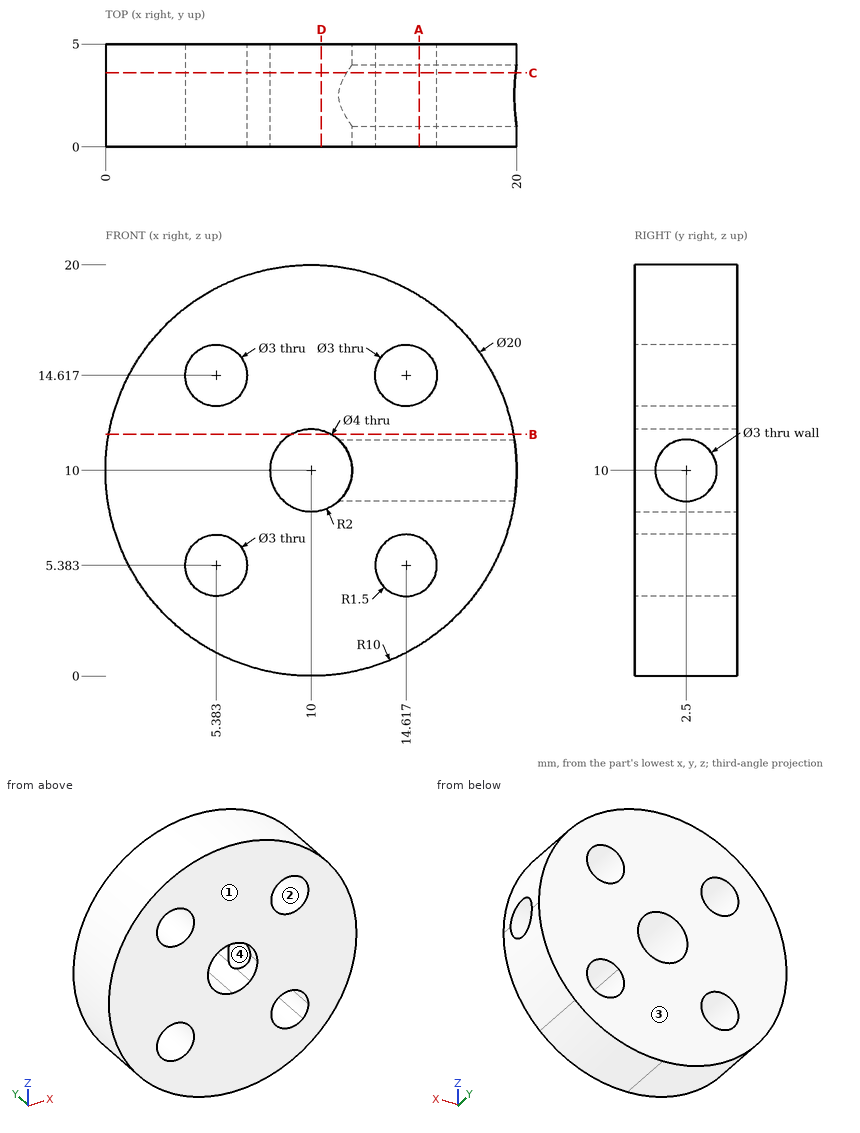
Can you work these out from the drawing? Everything is in mm from the part's minimum corner. Give positions to 0.01 mm unless a question says otherwise; leave off trailing zeros. Write each loop counter-clockwise with the first axis right and the second up, starting at its lowest first coordinate (ties: lowest second). Pieces come first, ordered by that corner, then holes. Notation, with made-up numbers: (64, 64) -> (90, 64) arc R18 cw to (90, 96) -> close; hole circle Ø8 at (40, 66.5). An arc over 180 degrees is marked (long way). Write each question's results on one line, items separated by ' | '. Start each with the question number.
Q1. Suppose I cut it at A-A, the plane x = 15.25. List the corners of the cut face in (y, z) for me.
Q2. We'd pull the mould along Y, two halves only. Please class the marked faces 1, 2, 3 and 4: +Y half, -Y half, draft (parallel to the pull), parting line (faces both ways), or undercut.
Q3. Suppose I cut it at B-B, the plane z = 11.75. List the corners of the cut face in (x, y) for me (1 decimal).
Q4. I'm going to push flat-ended pins straight in: pin 1 Ø2.5 at (x, z) = (10, 10) entering from -Y; pin 2 Ø1 at (y, z) = (3, 12.5) entering from -X; pin 3 Ø1 at (y, z) = (0.5, 4) entering from -X; pin 4 Ø1 at (x, y) = (17, 3) entering from +Z. Where does each tip first touch, or does it pass through?
Q5. Suppose I cut it at C-C, the plane y = 3.6. List the corners of the cut face in (x, z) for me (1 decimal), and give its area (3 significant figures).
Q6. I need wall thicknesses on probe 1 along Z at (x, y) = (5.5, 4); probe 2 along X at (y, z) = (1.85, 13.25) (1 decimal); probe 3 along Z at (x, y) = (9, 2.1). Which ranges of each line are inside material? Lowest first, please.
Q7. Suppose I cut it at D-D, the plane x = 10.5. List the corners of the cut face in (y, z) for me.
Outcome:
1) outline: (0, 1.49) -> (5, 1.49) -> (5, 4.02) -> (0, 4.02) -> close; (0, 6.74) -> (5, 6.74) -> (5, 13.26) -> (0, 13.26) -> close; (0, 15.98) -> (5, 15.98) -> (5, 18.51) -> (0, 18.51) -> close; hole circle Ø3 at (2.5, 10)
2) face 1: -Y half | face 2: draft | face 3: +Y half | face 4: undercut
3) outline: (0.2, 0) -> (9, 0) -> (9, 5) -> (0.2, 5) -> close; (11, 0) -> (19.8, 0) -> (19.8, 5) -> (11, 5) -> close
4) pin 1: through | pin 2: x = 0.2 | pin 3: x = 1.65 | pin 4: z = 17.6
5) outline: (11.7, 9) arc R2 cw (long way) to (11.7, 11) -> (19.9, 11) arc R10 ccw (long way) to (19.9, 9) -> close; hole circle Ø3 at (5.4, 5.4); hole circle Ø3 at (5.4, 14.6); hole circle Ø3 at (14.6, 5.4); hole circle Ø3 at (14.6, 14.6) | area: 257 mm2
6) probe 1: 1.07 to 3.89, 6.88 to 13.12, 16.11 to 18.93 | probe 2: 0.5 to 4.8, 6 to 14, 15.2 to 19.5 | probe 3: 0.05 to 8.27, 11.73 to 19.95
7) outline: (0, 0.01) -> (5, 0.01) -> (5, 8.06) -> (0, 8.06) -> close; (0, 11.94) -> (5, 11.94) -> (5, 19.99) -> (0, 19.99) -> close
